```python
from build123d import *

# Parameters (mm, degrees)
F1_DEPTH = 12.1
F2_R     = 2
F3_W     = 12
F3_H     = 7.62
F4_DEPTH = 20
F5_R     = 2.5
F6_DEPTH = 33.782


with BuildPart() as f1:
    # F0 (on Top) → F1 (new body)
    with BuildSketch(Plane.XY):
        with BuildLine():
            Line((6, -25), (6, -13.747727))
            ThreePointArc((6, -13.747727), (0, 15), (-6, -13.747727))
            Line((-6, -13.747727), (-6, -25))
            Line((-6, -25), (0, -25))
            Line((0, -25), (6, -25))
        make_face()
    extrude(amount=F1_DEPTH)

    # F2
    f2_edges = [f1.edges().sort_by_distance(p)[0] for p in [
        (0, 15, 12.1),
        (6, -19.373864, 12.1),
        (-6, -19.373864, 12.1),
        (0, -25, 12.1),
        (0, 15, 0),
        (6, -19.373864, 0),
        (-6, -19.373864, 0),
        (0, -25, 0),
    ]]
    fillet(f2_edges, radius=F2_R)

    # F3 (on face) → F4 (cut)
    with BuildSketch(Plane.XZ.offset(25)):
        with Locations((0, 6.05)):
            Rectangle(F3_W, F3_H)
    extrude(amount=-F4_DEPTH, mode=Mode.SUBTRACT)

    # F5 (on face) → F6 (cut)
    with BuildSketch(Plane.XZ.offset(5)):
        with Locations((0, 6.05)):
            Circle(F5_R)
    extrude(amount=-F6_DEPTH, mode=Mode.SUBTRACT)


solid = f1.part
```
Read the model definition and answer for the solid it produces. Units are mm, in the model's axes. A direction names the side the tool comes from. Give positions to 0.01 mm unless a question says otherwise; leave off trailing zeros. Loops run counter-clockwise (first coordinate to the right, second up) from the corner with the lowest first, then second, coordinate; pieces in that order, holes last.
Item 1: Find the intervals of material crossed by line 1 along Z through (x, y) = (0, 10.25); line 2 along Z through (x, y) = (-5, -6.5); line 3 along X through (y, z) = (-0.5, 6.05), in increasing order.
Item 2: The part is cut by section B-B (x = 0). Write down the section's boundary in (y, z).
Item 3: The part is cut by section A-A (y = -19). Write down the section's boundary in (x, z), and give its area (3 significant figures).
Item 4: The part is cut by section C-C (z = 6.05). Write down the section's boundary in (x, y).
Item 5: The part is cut by section D-D (z = 2.75). Write down the section's boundary in (x, y), and give its area (3 significant figures).
Item 6: The mould has two halves that part along X. Classify faces 1 (the cylindrical face through (5.43, -18.6, 0.6)), 2 (the flat face through (0, -15, 2.24)), 3 (the cylindrical face through (0.08, -24.43, 11.5)): released by +X, released by -X, zero draft, split by the parting line, or undercut.
Item 7: Each of these flat-tipped pins is pushed along its axis until it touches: pin 1 Ø4 at (y, z) = (-13, 5.5) entering from +X; pin 2 Ø3 at (x, z) = (0, 6.05) entering from +Y; pin 3 Ø5 at (x, z) = (9.5, 2.5) entering from +Y; pin 4 Ø4 at (x, z) = (-9.5, 6.5) entering from +Y. Where does it stop, or does it pass through?
Item 8: For faces 4 (the cylindrical face through (-5.43, -18.77, 11.5)), 5 (the cylindrical face through (-5.43, -18.77, 0.6)), 6 (the cylindrical face through (5.43, -18.6, 11.5)), 7 (the flat face through (0, -15, 9.86)), 8 (the flat face through (0, -1, 12.1)), determine the directions among +Z, -Z, +X, -X, +Y, -Y from which every point of the face is accessible in a straight line to the end or side of a thin tool.
Taken from the geometry:
1. line 1: z = 0 to 3.55, 8.55 to 12.1
1. line 2: z = 0 to 2.24, 9.86 to 12.1
1. line 3: x = -14.99 to -2.5, 2.5 to 14.99
2. outline: (-25, 2) arc R2 ccw to (-23, 0) - (13, 0) arc R2 ccw to (15, 2) - (15, 3.55) - (-5, 3.55) - (-5, 2.24) - (-25, 2.24) - close; (-25, 9.86) - (-5, 9.86) - (-5, 8.55) - (15, 8.55) - (15, 10.1) arc R2 ccw to (13, 12.1) - (-23, 12.1) arc R2 ccw to (-25, 10.1) - close
3. outline: (-6, 2) arc R2 ccw to (-4, 0) - (4, 0) arc R2 ccw to (6, 2) - (6, 2.24) - (-6, 2.24) - close; (-6, 9.86) - (6, 9.86) - (6, 10.1) arc R2 ccw to (4, 12.1) - (-4, 12.1) arc R2 ccw to (-6, 10.1) - close
3. area: 50.3 mm2
4. outline: (-6, -13.75) - (-6, -5) - (-2.5, -5) - (-2.5, 14.79) arc R15 ccw to start; (2.5, -5) - (6, -5) - (6, -13.75) arc R15 ccw to (2.5, 14.79) - close
5. outline: (-6, -13.75) - (-6, -5) - (6, -5) - (6, -13.75) arc R15 ccw (long way) to start
5. area: 592 mm2
6. face 1: released by +X
6. face 2: undercut
6. face 3: zero draft
7. pin 1: stops at x = 10.2
7. pin 2: passes through
7. pin 3: stops at y = 13.27
7. pin 4: stops at y = 12.99
8. face 4: +Z, -X, -Y
8. face 5: -Z, -X, -Y
8. face 6: +Z, +X, -Y
8. face 7: -Y
8. face 8: +Z, +X, -X, +Y, -Y
